Read the model definition and answer for the solid it produces. Units are mm, in the model's axes. Give positions to 0.01 mm unless a question says otherwise; leave off trailing zeros. Write each loop counter-clockwise with the first axis right and the second up, starting at its lowest first coordinate (ties: lowest second). Pieces come first, ordered by that corner, then holes. Notation, with made-up numbers: (68, 84) -> (101, 84) arc R19 ccw to (101, 97) -> close; hole circle Ø10 at (13, 69.5). An arc over 180 degrees is marked (long way). Answer as CSV lines item,"result". Start each with the question number.
1. For a pull along X with two mould halves and no side action, classify faces 1 (the cylindrical face through (-25.379, 48.794, 3.318)), 2 (the conical face through (49.99, -2.2, 234.65)), 3 (the flat face through (45, -24, 237.5)) as pulls with the +X half, pulls with the -X half, needs draft (parallel to the pull), parting line crosses it, or undercut.
2. The part is cut by section A-A, the plane z = 176. Determine the outline of the cut face in (x, y), and give its area (3 significant figures).
3. Given pin 1 (2 mm diameter, centred on x = 3, z = 158.5, fed in from +Y); pin 2 (5 mm diameter, centred on y = -8, z = 159, fed in from -X); pin 3 (1 mm diameter, centred on x = 41.5, z = 145.5, fed in from +Y), each flat-ended and moving along its own axis, determine where each tip first touches the part or whether it passes through.
4. Find the intervals of material crossed by line 1 (Y direction, x = 0, z = 53); line 2 (Y direction, x = -31.5, z = 37.5); line 3 (X direction, y = -30.5, z = 99.5), in increasing order.
from build123d import *
from OCP.BRepFilletAPI import BRepFilletAPI_MakeChamfer

# Parameters (mm, degrees)
SKETCH1_R               = 55
SKETCH1_R_2             = 50
TUBE_BODY_DEPTH         = 237.5
BORESINK_LEADIN_SIZE    = 0.8
BORESINK_LEADIN_SIZE2   = 3
BORESINK_LEADIN_2_SIZE  = 0.8
BORESINK_LEADIN_2_SIZE2 = 3
OD_EDGE_BREAK_SIZE      = 0.5


with BuildPart() as part:
    # Sketch1 → Tube Body (new, symmetric)
    with BuildSketch(Plane.XY):
        with Locations(Location((0, 0, 0), (0, 0, 180))):
            Circle(SKETCH1_R)
        with Locations(Location((0, 0, 0), (0, 0, 180))):
            Circle(SKETCH1_R_2, mode=Mode.SUBTRACT)
    extrude(amount=TUBE_BODY_DEPTH, both=True)

    # Boresink_Leadin: one chamfer whose edges measure the first distance from different faces: ONE call of the kernel's chamfer builder (chamfer() names one face for all edges)
    boresink_leadin_edges_1 = [part.edges().sort_by_distance(p)[0] for p in [
        (50, 0, -237.5),
    ]]
    boresink_leadin_side_1 = [part.faces().sort_by_distance(p)[0] for p in [
        (50, 0, 0),
    ]]
    boresink_leadin_edges_2 = [part.edges().sort_by_distance(p)[0] for p in [
        (50, 0, 237.5),
    ]]
    boresink_leadin_side_2 = [part.faces().sort_by_distance(p)[0] for p in [
        (53.444365081, 0, 237.5),
    ]]
    boresink_leadin = BRepFilletAPI_MakeChamfer(part.part.solid().wrapped)
    for e in boresink_leadin_edges_1:
        boresink_leadin.Add(BORESINK_LEADIN_SIZE, BORESINK_LEADIN_SIZE2, e.wrapped, boresink_leadin_side_1[0].wrapped)  # the first distance lies on this face
    for e in boresink_leadin_edges_2:
        boresink_leadin.Add(BORESINK_LEADIN_SIZE, BORESINK_LEADIN_SIZE2, e.wrapped, boresink_leadin_side_2[0].wrapped)  # the first distance lies on this face
    add(Compound.cast(boresink_leadin.Shape()), mode=Mode.REPLACE)

    # Boresink_Leadin 2
    boresink_leadin_2_edges = [part.edges().sort_by_distance(p)[0] for p in [
        (50, 0, -236.7),
    ]]
    boresink_leadin_2_side = [part.faces().sort_by_distance(p)[0] for p in [
        (51.5, 0, -237.1),
    ]]
    chamfer(boresink_leadin_2_edges, length=BORESINK_LEADIN_2_SIZE, length2=BORESINK_LEADIN_2_SIZE2, reference=boresink_leadin_2_side[0])

    # OD_Edge_Break
    od_edge_break_edges = [part.edges().sort_by_distance(p)[0] for p in [
        (55, 0, -237.5),
        (55, 0, 237.5),
    ]]
    chamfer(od_edge_break_edges, length=OD_EDGE_BREAK_SIZE)


solid = part.part
Results found:
1,face 1,"parting line crosses it"
1,face 2,"undercut"
1,face 3,"needs draft"
2,outline,"circle Ø110 at (0, 0); hole circle Ø100 at (0, 0)"
2,area,"1,650 mm²"
3,pin 1,"stops at y = 54.96"
3,pin 2,"stops at x = -54.72"
3,pin 3,"stops at y = 36.66"
4,line 1,"y = -55 to -50, 50 to 55"
4,line 2,"y = -45.09 to -38.83, 38.83 to 45.09"
4,line 3,"x = -45.77 to -39.62, 39.62 to 45.77"
